from build123d import *

# Parameters (mm, degrees)
SKETCH1_W                                         = 304.8
SKETCH1_H                                         = 254
BOSS_EXTRUDE1_DEPTH                               = 6.604
FILLET1_R                                         = 12.7
SKETCH6_W                                         = 50.8
SKETCH6_H                                         = 101.6
SKETCH6_W_2                                       = 44.45
SKETCH6_H_2                                       = 63.5
SKETCH6_W_3                                       = 38.1
SKETCH6_H_3                                       = 60.198
SKETCH6_W_4                                       = 120.65
SKETCH6_H_4                                       = 66.04
CUT_EXTRUDE1_DEPTH                                = 7.62
CUT_EXTRUDE2_DEPTH                                = 120.65
CUT_EXTRUDE3_DEPTH                                = 95.25
CUT_EXTRUDE4_DEPTH                                = 9.652
CSK_FOR_8_FLAT_HEAD_MACHINE_SCREW_100_D           = 4.9149
CSK_FOR_8_FLAT_HEAD_MACHINE_SCREW_100_DEPTH       = 10.668
CSK_FOR_8_FLAT_HEAD_MACHINE_SCREW_100_CSINK_D     = 8.4328
CSK_FOR_8_FLAT_HEAD_MACHINE_SCREW_100_CSINK_ANGLE = 100
CSK_FOR_8_FLAT_HEAD_MACHINE_SCREW_100_TIP         = 1.476584928


with BuildPart() as part:
    # Sketch1 → Boss-Extrude1 (new body)
    with BuildSketch(Plane.XY):
        Rectangle(SKETCH1_W, SKETCH1_H)
    extrude(amount=BOSS_EXTRUDE1_DEPTH)

    # Fillet1
    fillet1_edges = [part.edges().sort_by_distance(p)[0] for p in [
        (-152.4, 127, 3.302),
        (152.4, 127, 3.302),
        (152.4, -127, 3.302),
        (-152.4, -127, 3.302),
    ]]
    fillet(fillet1_edges, radius=FILLET1_R)

    # Sketch6 → Cut-Extrude1 (cut)
    with BuildSketch(Plane.XY.offset(6.604)):
        with Locations((-95.25, 43.688)):
            Rectangle(SKETCH6_W, SKETCH6_H)
        with Locations((0, 69.85)):
            Rectangle(SKETCH6_W_2, SKETCH6_H_2)
        with Locations((-101.6, -63.373)):
            Rectangle(SKETCH6_W_3, SKETCH6_H_3)
        with Locations((95.25, 43.688)):
            Rectangle(SKETCH6_W, SKETCH6_H)
        with Locations((78.105, -66.04)):
            Rectangle(SKETCH6_W_4, SKETCH6_H_4)
    extrude(amount=-CUT_EXTRUDE1_DEPTH, mode=Mode.SUBTRACT)

    # Sketch9 → Cut-Extrude2 (cut)
    with BuildSketch(Plane.ZY.offset(152.4)):
        with BuildLine():
            Line((6.604, 55.626), (6.604, 33.628954744))
            ThreePointArc((6.604, 33.628954744), (0.254, 44.627477372), (6.604, 55.626))
        make_face()
    cut_extrude2 = extrude(amount=-CUT_EXTRUDE2_DEPTH, mode=Mode.SUBTRACT)

    # Mirror1: Cut-Extrude2 across plane
    add(cut_extrude2.mirror(Plane(origin=(0, 0, 0), x_dir=(0, 0, 1), z_dir=(1, 0, 0))), mode=Mode.SUBTRACT)

    # Sketch10 → Cut-Extrude3 (cut)
    with BuildSketch(Plane.ZY.offset(152.4)):
        with BuildLine():
            Line((6.604, -52.678954744), (6.604, -74.676))
            ThreePointArc((6.604, -74.676), (0.254, -63.677477372), (6.604, -52.678954744))
        make_face()
    extrude(amount=-CUT_EXTRUDE3_DEPTH, mode=Mode.SUBTRACT)

    # Sketch11 → Cut-Extrude4 (cut)
    with BuildSketch(Plane.ZY.offset(-22.225)):
        with BuildLine():
            Line((6.604, 72.898), (6.604, 66.548))
            ThreePointArc((6.604, 66.548), (3.429, 69.723), (6.604, 72.898))
        make_face()
    cut_extrude4 = extrude(amount=-CUT_EXTRUDE4_DEPTH, mode=Mode.SUBTRACT)

    # Mirror2: Cut-Extrude4 across plane
    add(cut_extrude4.mirror(Plane(origin=(0, 0, 0), x_dir=(0, 0, 1), z_dir=(1, 0, 0))), mode=Mode.SUBTRACT)

    # CSK for #8 Flat Head Machine Screw (100)1
    with Locations(Plane(origin=(0, 0, 0), x_dir=(-1, 0, 0), z_dir=(0, 0, -1))):
        with Locations((-139.7, 114.3), (139.7, 114.3), (139.7, -114.3), (-139.7, -114.3)):
            CounterSinkHole(CSK_FOR_8_FLAT_HEAD_MACHINE_SCREW_100_D / 2, CSK_FOR_8_FLAT_HEAD_MACHINE_SCREW_100_CSINK_D / 2, depth=CSK_FOR_8_FLAT_HEAD_MACHINE_SCREW_100_DEPTH, counter_sink_angle=CSK_FOR_8_FLAT_HEAD_MACHINE_SCREW_100_CSINK_ANGLE)
            with Locations((0, 0, -(CSK_FOR_8_FLAT_HEAD_MACHINE_SCREW_100_DEPTH + CSK_FOR_8_FLAT_HEAD_MACHINE_SCREW_100_TIP / 2))):  # 118° drill point
                Cone(0, CSK_FOR_8_FLAT_HEAD_MACHINE_SCREW_100_D / 2, CSK_FOR_8_FLAT_HEAD_MACHINE_SCREW_100_TIP, mode=Mode.SUBTRACT)


solid = part.part
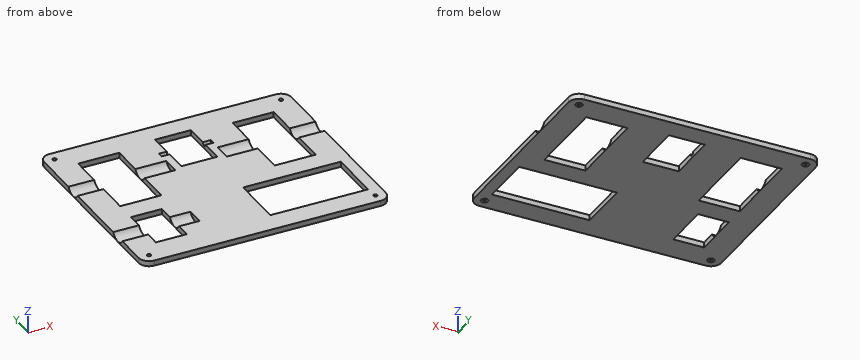
The listing builds one solid part. Answer for the finished solid, in the listing's coordinates (mm). Round coordinates to 2 decimals unless told otherwise and drop trailing zeros. Order: outer loops, then holes, each group sorted by start corner. A loop starts at its lowest first (then second) coordinate and runs counter-clockwise, first axis right, second up. Notation, with made-up numbers: M 72,7.5 L 103,7.5 A22 ccw 103,13.5 Z; hole C 20,59.25 d1. An arc over 180 degrees is marked long. Answer in a Markdown table with one row per item. Add a question column.
1) The part is cut by section C-C on x = -44.5. Determine the outline of the cut face in (y, z), plus the area to 3 significant figures.
2) Flat-ended cylindrical pins translate along their axes: pin 1 Ø3 at (y, z) = (39.5, 3.5) entering from -X; pin 2 Ø3 at (x, y) = (-139.7, -114.3) entering from -Z; pin 3 Ø6.5 at (x, y) = (139.7, 114.3) entering from +Z. Find the tip coordinate at first contact, or state that the pin passes through.
3) The part is cut by section B-B on y = -78. Determine the outline of the cut face in (x, z).
4) The part is cut by section D-D on y = 16.5. Determine the outline of the cut face in (x, z).
5) The part is cut by section A-A on y = 89. Determine the outline of the cut face in (x, z) (3 decimals).
6) Consider line 1 along X through (y, z) = (-34.5, 5); line 2 along Y through (x, z) = (110, 2.75); line 3 along X through (y, z) = (11, 1). Determine where each line is inside the solid, lowest interval first. Write a range as from..to.
Findings below:
| question | item | result |
|---|---|---|
| 1 | outline | M -127,0 L 127,0 L 127,6.6 L 55.63,6.6 A12.7 cw 33.63,6.6 L -127,6.6 Z |
| 1 | area | 1,580 mm² |
| 2 | pin 1 | stops at x = -31.75 |
| 2 | pin 2 | passes through |
| 2 | pin 3 | stops at z = 6.6 |
| 3 | outline | M -152.4,0 L -120.65,0 L -120.65,6.6 L -152.4,6.6 Z; M -82.55,0 L 17.78,0 L 17.78,6.6 L -82.55,6.6 Z; M 138.43,0 L 152.4,0 L 152.4,6.6 L 138.43,6.6 Z |
| 4 | outline | M -152.4,0 L -120.65,0 L -120.65,6.6 L -152.4,6.6 Z; M -69.85,0 L 69.85,0 L 69.85,6.6 L -69.85,6.6 Z; M 120.65,0 L 152.4,0 L 152.4,6.6 L 120.65,6.6 Z |
| 5 | outline | M -152.4,0 L -120.65,0 L -120.65,6.604 L -152.4,6.604 Z; M -69.85,0 L -22.225,0 L -22.225,6.604 L -69.85,6.604 Z; M 22.225,0 L 69.85,0 L 69.85,6.604 L 22.225,6.604 Z; M 120.65,0 L 152.4,0 L 152.4,6.604 L 120.65,6.604 Z |
| 6 | line 1 | x = -152.4..-120.65, -82.55..17.78, 138.43..152.4 |
| 6 | line 2 | y = -127..-99.06, -33.02..-7.11, 94.49..127 |
| 6 | line 3 | x = -152.4..-120.65, -69.85..69.85, 120.65..152.4 |
